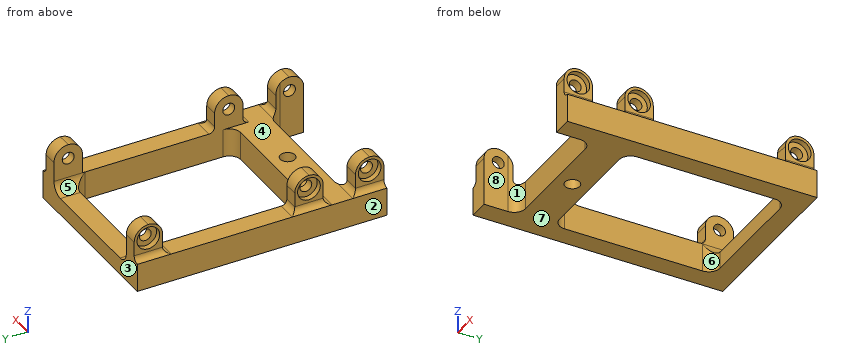
```python
from build123d import *

# Parameters (mm, degrees)
SKETCH2_W             = 3.5
SKETCH2_H             = 44
BOSS_EXTRUDE1_DEPTH   = 5
BOSS_EXTRUDE1_2_DEPTH = 5
SKETCH3_W             = 30
SKETCH3_H             = 3.5
BOSS_EXTRUDE2_DEPTH   = 3
SKETCH4_W             = 2.5
SKETCH4_H             = 5
BOSS_EXTRUDE3_DEPTH   = 6
SKETCH5_R             = 1.05
CUT_EXTRUDE1_DEPTH    = 39.026306684
FILLET1_R             = 2.5
FILLET2_R             = 2
SKETCH6_W             = 23
SKETCH6_H             = 6
SKETCH6_R             = 1.3
BOSS_EXTRUDE4_DEPTH   = 5
FILLET3_R             = 2
SKETCH7_R             = 2
CUT_EXTRUDE2_DEPTH    = 1
FILLET4_R             = 1


with BuildPart() as part:
    # Sketch2 → Boss-Extrude1 (new body)
    with BuildSketch(Plane.XY):
        with Locations((-13.25, 0)):
            Rectangle(SKETCH2_W, SKETCH2_H)
    extrude(amount=BOSS_EXTRUDE1_DEPTH)



with BuildPart() as body_2:
    # Sketch2 → Boss-Extrude1 2 (new body)
    with BuildSketch(Plane.XY):
        with Locations((13.25, 0)):
            Rectangle(SKETCH2_W, SKETCH2_H)
    extrude(amount=BOSS_EXTRUDE1_2_DEPTH)


with BuildPart() as part_1:
    add(part.part)

    add(body_2.part)  # Boss-Extrude2 merges body 2
    # Sketch3 → Boss-Extrude2 (add)
    with BuildSketch(Plane(origin=(0, 0, 0), x_dir=(-1, 0, 0), z_dir=(0, 0, -1))):
        with Locations((0, 20.25)):
            Rectangle(SKETCH3_W, SKETCH3_H)
    extrude(amount=-BOSS_EXTRUDE2_DEPTH)

    # Sketch4 → Boss-Extrude3 (add)
    with BuildSketch(Plane.XY.offset(5)):
        with Locations((-12.75, 19.5)):
            Rectangle(SKETCH4_W, SKETCH4_H)
        with Locations((-12.75, -8.8)):
            Rectangle(SKETCH4_W, SKETCH4_H)
        with Locations((-12.75, -19.5)):
            Rectangle(SKETCH4_W, SKETCH4_H)
        with Locations((12.75, -19.5)):
            Rectangle(SKETCH4_W, SKETCH4_H)
        with Locations((12.75, -8.8)):
            Rectangle(SKETCH4_W, SKETCH4_H)
        with Locations((12.75, 19.5)):
            Rectangle(SKETCH4_W, SKETCH4_H)
    extrude(amount=BOSS_EXTRUDE3_DEPTH)

    # Sketch5 → Cut-Extrude1 (cut, through all)
    with BuildSketch(Plane.ZY.offset(14)):
        with Locations((8.5, 19.5)):
            Circle(SKETCH5_R)
        with Locations((8.5, -8.8)):
            Circle(SKETCH5_R)
        with Locations((8.5, -19.5)):
            Circle(SKETCH5_R)
    extrude(amount=-CUT_EXTRUDE1_DEPTH, mode=Mode.SUBTRACT)

    # Fillet1
    fillet1_edges = [part_1.edges().sort_by_distance(p)[0] for p in [
        (12.75, -17, 11),
        (12.75, -22, 11),
        (12.75, -6.3, 11),
        (12.75, -11.3, 11),
        (-12.75, -22, 11),
        (-12.75, -17, 11),
        (-12.75, -11.3, 11),
        (-12.75, -6.3, 11),
        (-12.75, 17, 11),
        (-12.75, 22, 11),
        (12.75, 22, 11),
        (12.75, 17, 11),
    ]]
    fillet(fillet1_edges, radius=FILLET1_R - 0.0001)  # a hair under: the kernel refuses the full size

    # Fillet2
    fillet2_edges = [part_1.edges().sort_by_distance(p)[0] for p in [
        (-11.5, 20.25, 3),
        (-11.5, 18.5, 1.5),
        (11.5, 18.5, 1.5),
        (11.5, 20.25, 3),
    ]]
    fillet(fillet2_edges, radius=FILLET2_R - 0.0001)  # a hair under: the kernel refuses the full size

    # Sketch6 → Boss-Extrude4 (add)
    with BuildSketch(Plane(origin=(0, 0, 0), x_dir=(-1, 0, 0), z_dir=(0, 0, -1))):
        with Locations((0, -12.8)):
            Rectangle(SKETCH6_W, SKETCH6_H)
        with Locations((0, -12.8)):
            Circle(SKETCH6_R, mode=Mode.SUBTRACT)
    extrude(amount=-BOSS_EXTRUDE4_DEPTH)

    # Fillet3
    fillet3_edges = [part_1.edges().sort_by_distance(p)[0] for p in [
        (-11.5, -9.8, 2.5),
        (-11.5, -15.8, 2.5),
        (11.5, -15.8, 2.5),
        (11.5, -9.8, 2.5),
    ]]
    fillet(fillet3_edges, radius=FILLET3_R)

    # Sketch7 → Cut-Extrude2 (cut)
    with BuildSketch(Plane.ZY.offset(14)):
        with Locations((8.5, 19.5)):
            Circle(SKETCH7_R)
        with Locations((8.5, -8.8)):
            Circle(SKETCH7_R)
        with Locations((8.5, -19.5)):
            Circle(SKETCH7_R)
    cut_extrude2 = extrude(amount=-CUT_EXTRUDE2_DEPTH, mode=Mode.SUBTRACT)

    # Mirror1: Cut-Extrude2 across plane
    add(cut_extrude2.mirror(Plane(origin=(0, 0, 0), x_dir=(0, 0, 1), z_dir=(1, 0, 0))), mode=Mode.SUBTRACT)

    # Fillet4
    fillet4_edges = [part_1.edges().sort_by_distance(p)[0] for p in [
        (12.75, -11.3, 5),
        (-12.75, -11.3, 5),
        (-12.75, 17, 5),
        (14, -19.5, 5),
        (14, -8.8, 5),
        (14, 19.5, 5),
        (-12.75, -6.3, 5),
        (-12.666515139, -17, 5),
        (-14, -19.5, 5),
        (-14, -8.8, 5),
        (12.666515139, -17, 5),
        (12.75, -6.3, 5),
        (-14, 19.5, 5),
    ]]
    fillet(fillet4_edges, radius=FILLET4_R - 0.0001)  # a hair under: the kernel refuses the full size


solid = part_1.part
```
Input: part model. Units: mm. Frame: model coordinates. Face numbers are marked on the shaded views. A direction names the side the tool comes from. Coordinates: 2 decimals unless noted, no trailing zeros. Loops run counter-clockwise (first coordinate to the right, second up) from the corner with the lowest first, then second, coordinate; pieces in that order, holes last.
Q1. Contact query for flat-ended pins moving along their axis: pin 1 (3 mm diameter, centred on y = -8, z = 9, fed in from +X); pin 2 (1.7 mm diameter, centred on y = 19.5, z = 8.5, fed in from +X); pin 3 (1.2 mm diameter, centred on y = -19, z = 8, fed in from -X); pin 4 (1.3 mm diameter, centred on y = -19.5, z = 6.5, fed in from -X). Output: stop coordinate, or through.
Results are:
pin 1: stops at x = 14
pin 2: passes through
pin 3: stops at x = -13
pin 4: stops at x = -14.01
Q2. Line query: line 1 along Y through (x, z) = (-12.5, 8.5); line 2 along Y through (x, z) = (-13.7, 8.5); line 3 along Y through (x, z) = (-9, 1). Output: solid intervals per line, ascending.
Results are:
line 1: y = -22 to -20.55, -18.45 to -17, -11.3 to -9.85, -7.75 to -6.3, 17 to 18.45, 20.55 to 22
line 2: y = -22 to -21.5, -17.5 to -17, -11.3 to -10.8, -6.8 to -6.3, 17 to 17.5, 21.5 to 22
line 3: y = -15.8 to -9.8, 18.5 to 22
Q3. Mould query, pull axis X, two halves, no side actions, for the marked faces 1, 2 and 3. Classes: +X half, -X half, draft (parallel to the pull), parting line (faces both ways), or undercut.
Results are:
face 1: undercut
face 2: -X half
face 3: draft
Q4. Section B-B, the plane x = 5. Return the cut outline in (y, z).
Results are:
outline: (-15.8, 0) - (-9.8, 0) - (-9.8, 5) - (-15.8, 5) - close; (18.5, 0) - (22, 0) - (22, 3) - (18.5, 3) - close
Q5. Section D-D, the plane z = 8. Give the number of separate pieces and of enclosed holes in the cut face, and give its area (3 significant figures).
Results are:
separate pieces: 12
enclosed holes: 0
area: 35.2 mm2
Q6. Set-up query: the marked faces 4, 5, 6, 7 and 8. Return all of +Z, -Z, +X, -X, +Y, -Y with unobstructed straight access to the full face (end or side cutting, diameter ignored); none if empty.
Results are:
face 4: +Z
face 5: +Z, +Y
face 6: +Z, -Z
face 7: -Z, +X, -X, +Y, -Y
face 8: +Z, -Z, -Y
Q7. Section C-C, the plane z = 0.5. Return the cut outline in (x, y), and give its area (3 significant figures).
Results are:
outline: (-15, -22) - (-11.5, -22) - (-11.5, -17.8) arc R2 cw to (-9.5, -15.8) - (9.5, -15.8) arc R2 cw to (11.5, -17.8) - (11.5, -22) - (15, -22) - (15, 22) - (-15, 22) - close; hole (-11.5, -7.8) arc R2 ccw to (-9.5, -9.8) - (9.5, -9.8) arc R2 ccw to (11.5, -7.8) - (11.5, 16.5) arc R2 ccw to (9.5, 18.5) - (-9.5, 18.5) arc R2 ccw to (-11.5, 16.5) - close; hole circle Ø2.6 at (0, -12.8)
area: 526 mm2
Q8. Section A-A, the plane y = 1. Return the cut outline in (x, z), and give its area (3 significant figures).
Results are:
outline: (-15, 0) - (-11.5, 0) - (-11.5, 5) - (-15, 5) - close; (11.5, 0) - (15, 0) - (15, 5) - (11.5, 5) - close
area: 35.0 mm2
